Could you check a few things on this model? Use its own coordinates, in mm. Give positions to 0.01 mm unless a question says otherwise; leave off trailing zeros. Loops run counter-clockwise (first coordinate to the right, second up) from the corner with the lowest first, then second, coordinate; pieces in that order, holes last. Notation, with made-up numbers: (53, 26) - (65, 26) arc R17 ccw to (65, 56) - close; hole circle Ø11 at (-8.5, 60). An arc over 180 degrees is marked (long way). Write each question's results on one line, items separated by ' | '. Start each with the question number.
1) I want a section at B-B, the plane y = 10. Count the separate pieces of the cut face and the enclosed holes in it, and give its area (3 significant figures).
2) I want a section at C-C, the plane x = 44. Write out the boundary of the cut face in (y, z), and give its area (3 significant figures).
3) If I drill on probe 1 along Z at (x, y) = (5.5, 3); probe 2 along Z at (x, y) = (7, 6); probe 3 along Z at (x, y) = (55.5, 10.5), over which ranges is the centre line in solid material (lowest first)? Write a range as [from, to].
4) I want a section at D-D, the plane z = -19. Write out the boundary of the cut face in (x, y), and give its area (3 significant figures).
5) I want a section at A-A, the plane z = -80.5. Write out the boundary of the cut face in (x, y).
6) I'm going to push flat-ended pins straight in: pin 1 (2 mm diameter, centred on x = 47, y = 8.5, fed in from +Z); pin 2 (3 mm diameter, centred on x = 31, y = 1.5, fed in from +Z); pin 3 (4.5 mm diameter, centred on x = 5.08, z = -5.4, fed in from -Y); pin 4 (6 mm diameter, centred on x = 30, y = 5.5, fed in from +Z). Where does each tip first touch, or does it pass through?
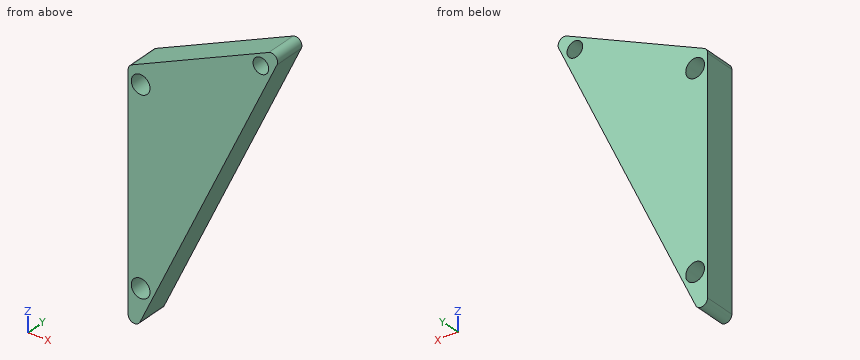
from build123d import *

# Parameters (mm, degrees)
BOSS_EXTRUDE1_DEPTH = 12.7
SKETCH2_R           = 3.81
SKETCH2_R_2         = 3.175
CUT_EXTRUDE1_DEPTH  = 124.712602834
FILLET1_R           = 2.54


with BuildPart() as part:
    # Sketch1 → Boss-Extrude1 (new body)
    with BuildSketch(Plane(origin=(0, 0, 0), x_dir=(1, 0, 0), z_dir=(0, 1, 0))):
        Polygon((0, 0), (0, 105.41), (63.5, -29.464), align=None)
    extrude(amount=BOSS_EXTRUDE1_DEPTH)

    # Sketch2 → Cut-Extrude1 (cut, through all)
    with BuildSketch(Plane.XZ):
        with Locations(Location((5.08, -82.347196418, 0), (0, 0, 270))):
            Circle(SKETCH2_R)
        with Locations(Location((5.08, -5.39556681, 0), (0, 0, 270))):
            Circle(SKETCH2_R)
        with Locations(Location((53.955653889, 20.261534242, 0), (0, 0, 270))):
            Circle(SKETCH2_R_2)
    extrude(amount=-CUT_EXTRUDE1_DEPTH, mode=Mode.SUBTRACT)

    # Fillet1
    fillet1_edges = [part.edges().sort_by_distance(p)[0] for p in [
        (0, 6.35, 0),
        (0, 6.35, -105.41),
        (63.5, 6.35, 29.464),
    ]]
    fillet(fillet1_edges, radius=FILLET1_R)


solid = part.part
Answers:
1) separate pieces: 1 | enclosed holes: 3 | area: 3,190 mm2
2) outline: (0, -11.95) - (12.7, -11.95) - (12.7, 20.42) - (0, 20.42) - close | area: 411 mm2
3) probe 1: z = [-93.73, -86.13], [-78.56, -9.18], [-1.61, 2.55] | probe 2: z = [-90.54, -85.64], [-79.06, -8.69], [-2.1, 3.25] | probe 3: z = [12.47, 17.49], [23.04, 25.75]
4) outline: (0, 0) - (40.68, 0) - (40.68, 12.7) - (0, 12.7) - close | area: 517 mm2
5) outline: (0, 0) - (1.75, 0) - (1.75, 12.7) - (0, 12.7) - close; (8.41, 0) - (11.73, 0) - (11.73, 12.7) - (8.41, 12.7) - close
6) pin 1: stops at z = 22.27 | pin 2: stops at z = 15.08 | pin 3: passes through | pin 4: stops at z = 15.31
